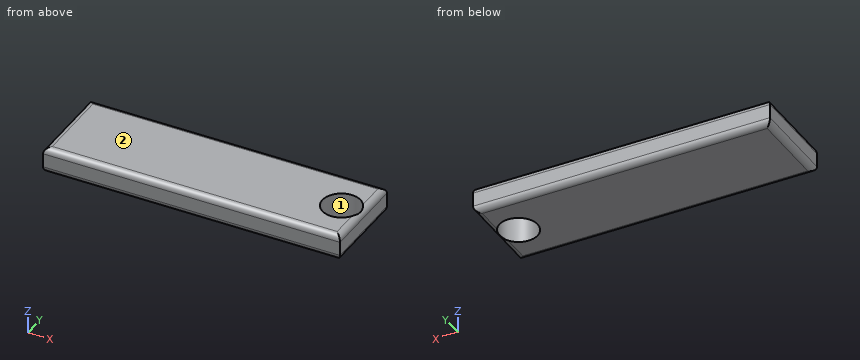
from build123d import *

# Parameters (mm, degrees)
SKETCH1_W           = 34.29
SKETCH1_H           = 10.16
SKETCH1_R           = 2.2
BOSS_EXTRUDE1_DEPTH = 3
FILLET1_R           = 0.7


with BuildPart() as part:
    # Sketch1 → Boss-Extrude1 (new body)
    with BuildSketch(Plane.XY):
        with Locations((17.145, 5.08)):
            Rectangle(SKETCH1_W, SKETCH1_H)
        with Locations((31.75, 5.08)):
            Circle(SKETCH1_R, mode=Mode.SUBTRACT)
    extrude(amount=BOSS_EXTRUDE1_DEPTH)

    # Fillet1
    # the kernel refuses this fillet: 0.7 mm, written as the material it takes off along each edge
    with BuildSketch(Plane(origin=(34.29, 11.91, 3), x_dir=(0, 0, -1), z_dir=(0, -1, 0)), Plane(origin=(0, -1.75, 3), x_dir=(0, 0, -1), z_dir=(0, 1, 0))) as fillet1_piece_1:
        with BuildLine():
            CenterArc((FILLET1_R, -FILLET1_R), FILLET1_R, 90, 90)
            Line((0, -FILLET1_R), (0, 0))
            Line((0, 0), (FILLET1_R, 0))
        make_face()
    extrude(amount=13.66, mode=Mode.SUBTRACT)
    with BuildSketch(Plane(origin=(-1.75, 10.16, 3), x_dir=(0, 0, -1), z_dir=(1, 0, 0)), Plane(origin=(36.04, 0, 3), x_dir=(0, 0, -1), z_dir=(-1, 0, 0))) as fillet1_piece_2:
        with BuildLine():
            CenterArc((FILLET1_R, -FILLET1_R), FILLET1_R, 90, 90)
            Line((0, -FILLET1_R), (0, 0))
            Line((0, 0), (FILLET1_R, 0))
        make_face()
    extrude(amount=37.79, mode=Mode.SUBTRACT)
    with BuildSketch(Plane(origin=(-1.75, 10.16, 0), x_dir=(0, 0, 1), z_dir=(1, 0, 0)), Plane(origin=(36.04, 0, 0), x_dir=(0, 0, 1), z_dir=(-1, 0, 0))) as fillet1_piece_3:
        with BuildLine():
            CenterArc((FILLET1_R, FILLET1_R), FILLET1_R, 180, 90)
            Line((0, FILLET1_R), (0, 0))
            Line((0, 0), (FILLET1_R, 0))
        make_face()
    extrude(amount=37.79, mode=Mode.SUBTRACT)
    with BuildSketch(Plane(origin=(34.29, 11.91, 0), x_dir=(0, 0, 1), z_dir=(0, -1, 0)), Plane(origin=(0, -1.75, 0), x_dir=(0, 0, 1), z_dir=(0, 1, 0))) as fillet1_piece_4:
        with BuildLine():
            CenterArc((FILLET1_R, FILLET1_R), FILLET1_R, 180, 90)
            Line((0, FILLET1_R), (0, 0))
            Line((0, 0), (FILLET1_R, 0))
        make_face()
    extrude(amount=13.66, mode=Mode.SUBTRACT)


solid = part.part
Here's how the part is built. I have some questions about the finished solid (model axes, mm). Face numbers are marked on the shaded views. Give positions to 0.01 mm unless a question says otherwise; leave off trailing zeros. Write each loop counter-clockwise with the first axis right and the second up, starting at its lowest first coordinate (ties: lowest second). Pieces come first, ordered by that corner, then holes. Notation, with made-up numbers: (-31.75, 72) -> (21.25, 72) arc R15 ccw to (21.25, 90) -> close; hole circle Ø8 at (25.25, -24). An arc over 180 degrees is marked (long way). Use one line per item in the form item = value. Start each with the question number.
1. Imagine slicing it at A-A on x = 31.75. List the corners of the cut face in (y, z) for me.
2. Imagine slicing it at D-D on y = 9.75. List the corners of the cut face in (x, z) for me, plus the area to 3 significant figures.
3. Imagine slicing it at B-B on y = 6.75. List the corners of the cut face in (x, z) for me.
4. Thinking about a two-plate mould opening in Y: for the marked faces 1 and 2, which applies, +Y half, -Y half, draft (parallel to the pull), parting line (faces both ways), or undercut?
5. Will this pin go through, and if not, where does the flat tip stop? pin 1 Ø3.5 at (x, y) = (31.75, 5.08) entering from -Z.
6. If I drill on L1, parallel to X at y = 5.08, z = 2.1; L2, parallel to Y at x = 31.75, z = 2.2; L3, parallel to Y at x = 30, z = 0.7, over which ranges is the centre line in solid material (lowest first)?
7. Imagine slicing it at C-C on z = 1.8. List the corners of the cut face in (x, y) for me.
Entries:
q1.outline = (0, 0.7) arc R0.7 ccw to (0.7, 0) -> (2.88, 0) -> (2.88, 3) -> (0.7, 3) arc R0.7 ccw to (0, 2.3) -> close; (7.28, 0) -> (9.46, 0) arc R0.7 ccw to (10.16, 0.7) -> (10.16, 2.3) arc R0.7 ccw to (9.46, 3) -> (7.28, 3) -> close
q2.outline = (0, 0.7) arc R0.7 ccw to (0.41, 0.06) -> (33.88, 0.06) arc R0.7 ccw to (34.29, 0.7) -> (34.29, 2.3) arc R0.7 ccw to (33.88, 2.94) -> (0.41, 2.94) arc R0.7 ccw to (0, 2.3) -> close
q2.area = 98.3 mm²
q3.outline = (0, 0.7) arc R0.7 ccw to (0.7, 0) -> (30.32, 0) -> (30.32, 3) -> (0.7, 3) arc R0.7 ccw to (0, 2.3) -> close; (33.18, 0) -> (33.59, 0) arc R0.7 ccw to (34.29, 0.7) -> (34.29, 2.3) arc R0.7 ccw to (33.59, 3) -> (33.18, 3) -> close
q4.face_1 = undercut
q4.face_2 = draft
q5.pin_1 = through
q6.L1 = 0 to 29.55, 33.95 to 34.29
q6.L2 = 0 to 2.88, 7.28 to 10.16
q6.L3 = 0 to 3.75, 6.41 to 10.16
q7.outline = (0, 0) -> (34.29, 0) -> (34.29, 10.16) -> (0, 10.16) -> close; hole circle Ø4.4 at (31.75, 5.08)
